Input: dimensioned drawing with shaded views. Units: mm. Origin: part minimum x, y, z. Round coordinates to 2 decimals unless told otherwise and drop trailing zeros. Loops run counter-clockwise (first coordinate to the right, second up) from the corner with the lowest first, then second, coordinate; pieces in that order, holes last.
Item 1: Pull-direction query (X, two-part tool) for the marked faces 1 and 2; classes: released by +X, released by -X, zero draft, split by the parting line, or undercut.
Item 2: Section query A-A on z = 1.35. Return loops of the section in (x, y).
Item 3: Section query C-C on x = 8.5. Return loops of the section in (y, z).
Item 4: First-contact query: P1, Ø0.8, axis at x = 6, z = 1, coming from the -Y side; P2, Ø0.8, axis at y = 8, z = 1, coming from the -X side; P3, Ø0.5, axis at y = 14.5, z = 1, coming from the -X side. Flat tips, straight axial feed; report the tip coordinate or a pass-through.
Item 5: Ray query, L1, parallel to X at y = 7.25, z = 0.8; L2, parallel to Z at x = 4, y = 10.5; L3, parallel to Y at x = 5, z = 0.55. Return the intervals inside material, ascending.
Item 6: Section query B-B on y = 7. Return loops of the section in (x, z).
Item 7: Section query D-D on y = 11. Return loops of the section in (x, z), then the cut area to 3 significant figures.
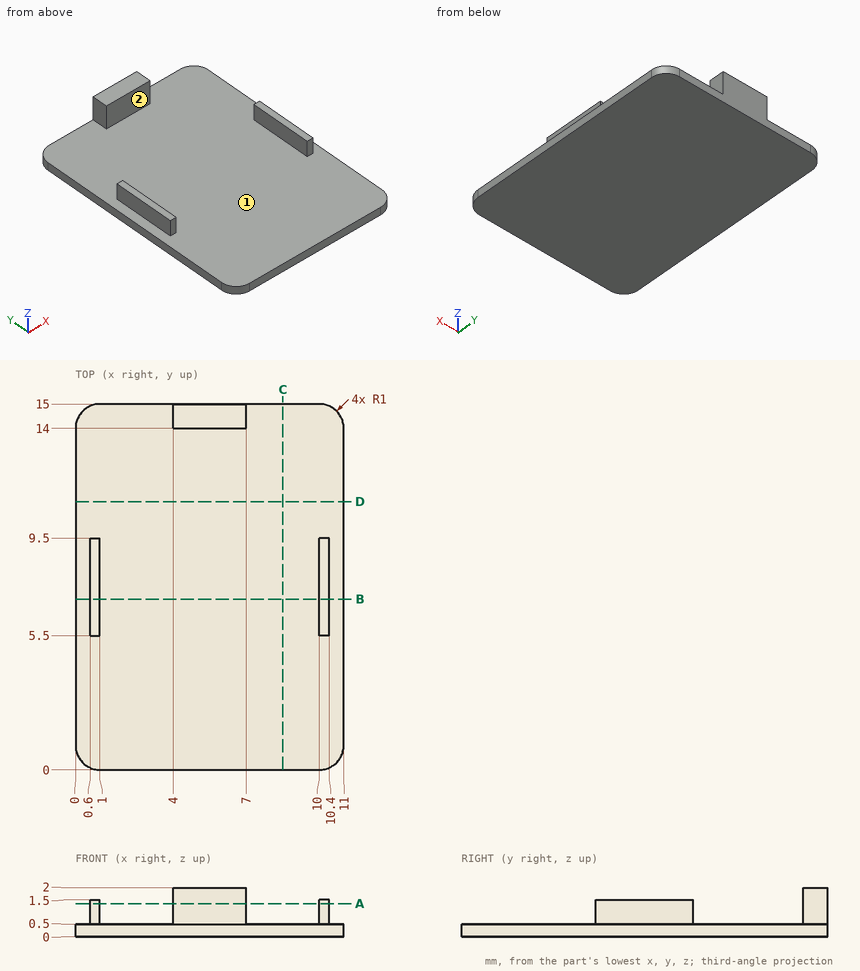
Data:
1. face 1: undercut
1. face 2: zero draft
2. outline: (0.6, 5.5) - (1, 5.5) - (1, 9.5) - (0.6, 9.5) - close; (4, 14) - (7, 14) - (7, 15) - (4, 15) - close; (10, 5.5) - (10.4, 5.5) - (10.4, 9.5) - (10, 9.5) - close
3. outline: (0, 0) - (15, 0) - (15, 0.5) - (0, 0.5) - close
4. P1: stops at y = 14
4. P2: stops at x = 0.6
4. P3: stops at x = 4
5. L1: x = 0.6 to 1, 10 to 10.4
5. L2: z = 0 to 0.5
5. L3: y = 14 to 15
6. outline: (0, 0) - (11, 0) - (11, 0.5) - (10.4, 0.5) - (10.4, 1.5) - (10, 1.5) - (10, 0.5) - (1, 0.5) - (1, 1.5) - (0.6, 1.5) - (0.6, 0.5) - (0, 0.5) - close
7. outline: (0, 0) - (11, 0) - (11, 0.5) - (0, 0.5) - close
7. area: 5.50 mm2
